Source: CAD feature listing. Evaluate the final solid. Frame: model axes, mm. A direction names the side the tool comes from. Give positions to 0.01 mm unless a question says otherwise; leave off trailing zeros. Order: outer loops, then holes, each group sorted by start corner. A loop starts at its lowest first (then second) coordinate and runs counter-clockwise, first axis right, second up. Notation, with made-up numbers: M 89.5,60.25 L 99.5,60.25 A8 ccw 99.5,69.25 Z; hole C 14.25,-33 d1. An arc over 180 degrees is marked long. Answer as a JSON object with one key per item and string values. Group by question number.
1. Set-up query: faces 1 (the flat face through (30, 0, 10)), 2 (the flat face through (0, -6.25, 2)), 3 (the cylindrical face through (21.514, 0.477, 18.028)). Return all of +Z, -Z, +X, -X, +Y, -Y with unobstructed straight access to the full face (end or side cutting, diameter ignored); none if empty.
2. Pull-direction query (Z, two-part tool) for faces 4 (the flat face through (0, 6.25, 2)), 5 (the flat face through (0, 11, 0)), 6 (the flat face through (0, 11, 4)); classes: +Z half, -Z half, draft (parallel to the pull), parting line (faces both ways), or undercut.
3. Section query B-B (z = 11.5). Output: boundary loops of the cut face in (x, y), plus the area to 3 significant figures.
4. Pin query (flat end, axial travel): P1, Ø1.9, axis at x = 20, y = 0, coming from the -Z side. Return the tip coordinate at first contact, or that it passes through.
5. Section query A-A (x = 20). Output: boundary loops of the cut face in (y, z).
6. Material intervals for L1, parallel to Z at x = -15, y = -21; L2, parallel to X at y = 14.5, z = 11; L3, parallel to Y at x = 20, z = 18.9, sorted ascending. Write a range as [from, to].
7. Section query D-D (y = 0). Output: boundary loops of the cut face in (x, z), plus the area to 3 significant figures.
8. Section query C-C (x = 28.5). Output: boundary loops of the cut face in (y, z).
from build123d import *

# Parameters (mm, degrees)
F0_W     = 60
F0_H     = 50
F0_W_2   = 23
F0_H_2   = 12.5
F0_R     = 1.5875
F1_DEPTH = 4
F0_W_3   = 4
F2_DEPTH = 20
F4_W     = 60
F4_H     = 50
F4_R     = 1.5875
F5_DEPTH = 4


with BuildPart() as f1:
    # F0 (on Top) → F1 (new body)
    with BuildSketch(Plane.XY):
        Rectangle(F0_W, F0_H)
        with Locations((0.25, 0)):
            Rectangle(F0_W_2, F0_H_2, mode=Mode.SUBTRACT)
        with Locations((20, 0)):
            Circle(F0_R, mode=Mode.SUBTRACT)
    extrude(amount=F1_DEPTH)

    # F0 (on Top) → F2 (join)
    with BuildSketch(Plane.XY):
        with Locations((-32, 0)):
            Rectangle(F0_W_3, F0_H)
        with Locations((32, 0)):
            Rectangle(F0_W_3, F0_H)
    extrude(amount=F2_DEPTH)

    # F4 (on offset) → F5 (join)
    with BuildSketch(Plane.XY.offset(20)):
        Rectangle(F4_W, F4_H)
        with Locations((20, 0)):
            Circle(F4_R, mode=Mode.SUBTRACT)
    extrude(amount=-F5_DEPTH)


solid = f1.part
Answer sheet:
{
 "1": {"face 1": "+Y, -Y", "face 2": "-Z", "face 3": "+Z, -Z"},
 "2": {"face 4": "draft", "face 5": "-Z half", "face 6": "undercut"},
 "3": {"outline": "M -34,-25 L -30,-25 L -30,25 L -34,25 Z; M 30,-25 L 34,-25 L 34,25 L 30,25 Z", "area": "400 mm^2"},
 "4": {"P1": "through"},
 "5": {"outline": "M -25,0 L -1.59,0 L -1.59,4 L -25,4 Z; M -25,16 L -1.59,16 L -1.59,20 L -25,20 Z; M 1.59,0 L 25,0 L 25,4 L 1.59,4 Z; M 1.59,16 L 25,16 L 25,20 L 1.59,20 Z"},
 "6": {"L1": "[0, 4], [16, 20]", "L2": "[-34, -30], [30, 34]", "L3": "[-25, -1.59], [1.59, 25]"},
 "7": {"outline": "M -34,0 L -11.25,0 L -11.25,4 L -30,4 L -30,16 L 18.41,16 L 18.41,20 L -34,20 Z; M 11.75,0 L 18.41,0 L 18.41,4 L 11.75,4 Z; M 21.59,0 L 34,0 L 34,20 L 21.59,20 L 21.59,16 L 30,16 L 30,4 L 21.59,4 Z", "area": "523 mm^2"},
 "8": {"outline": "M -25,0 L 25,0 L 25,4 L -25,4 Z; M -25,16 L 25,16 L 25,20 L -25,20 Z"}
}
